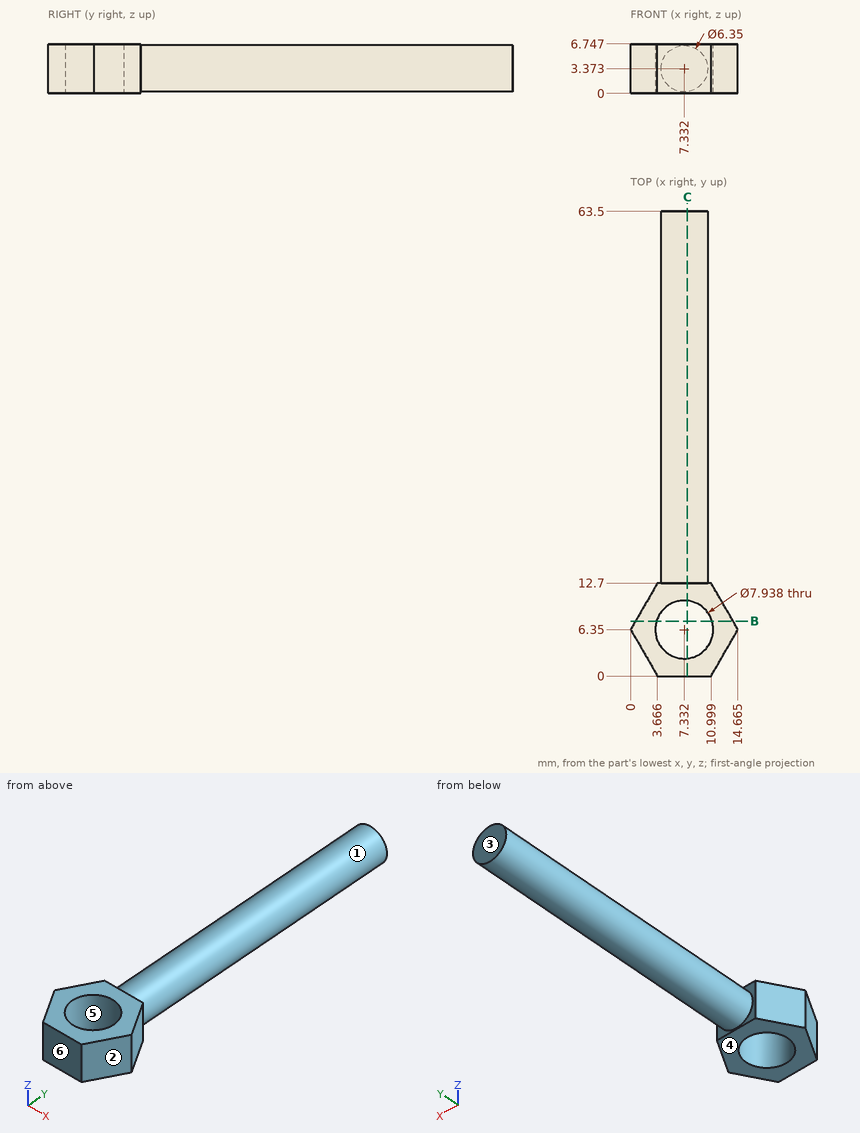
Study the drawing (mm; zero at the part's minimum x, y, z) and answer. A direction names the side the tool comes from. Coordinates: 2 decimals unless noted, no trailing zeros. Order: outer loops, then holes, each group sorted by start corner. A loop starts at its lowest first (then second) coordinate and runs counter-clockwise, first axis right, second up. Notation, with made-up numbers: (-33, 34) -> (-27, 34) arc R27 cw to (-27, 55) -> close; hole circle Ø3 at (44, 63.25). An arc over 180 degrees is marked (long way). Answer in a Markdown table with one row per item. Add a question column.
Item 1: Determine the mould class of the marked faces 3, 4, 5 and 6 for opening direction Y: +Y half, -Y half, draft (parallel to the pull), parting line (faces both ways), or undercut.
Item 2: Which of the six approach directions +Z, -Z, +X, -X, +Y, -Y give full straight-line access (tool end or side, diameter ignored) to the marked faces 1 and 2?
Item 3: Find section C-C (x = 7.75). Write down the section's boundary in (y, z).
Item 4: Find the intervals of material crossed by L1, parallel to Y at x = 6, z = 1; L2, parallel to Y at x = 9.5, z = 4.5 (1 decimal); L3, parallel to X at y = 14.5, z = 1.75 (1 decimal), in increasing order. Write a range as from..to.
Item 5: Find section B-B (y = 7.5). Write down the section's boundary in (x, z).
Item 6: Each of these flat-tipped pins is pushed along its axis until it touches: P1, Ø3, axis at x = 11, y = 15, coming from the +Z side (1 decimal); P2, Ø4, axis at x = 6, y = 46, coming from the -Z side. Where does it stop, or does it pass through?
Result set:
| question | item | result |
|---|---|---|
| 1 | face 3 | +Y half |
| 1 | face 4 | draft |
| 1 | face 5 | undercut |
| 1 | face 6 | -Y half |
| 2 | face 1 | +Y |
| 2 | face 2 | +Z, -Z, +X, -Y |
| 3 | outline | (0, 0) -> (2.4, 0) -> (2.4, 6.75) -> (0, 6.75) -> close; (10.3, 0) -> (12.7, 0) -> (12.7, 0.23) -> (63.5, 0.23) -> (63.5, 6.52) -> (12.7, 6.52) -> (12.7, 6.75) -> (10.3, 6.75) -> close |
| 4 | L1 | y = 0..2.61, 10.09..63.5 |
| 4 | L2 | y = 0..3, 9.7..63.5 |
| 4 | L3 | x = 4.6..10.1 |
| 5 | outline | (0.66, 0) -> (3.53, 0) -> (3.53, 6.75) -> (0.66, 6.75) -> close; (11.13, 0) -> (14, 0) -> (14, 6.75) -> (11.13, 6.75) -> close |
| 6 | P1 | stops at z = 5.7 |
| 6 | P2 | stops at z = 0.2 |
